Geometry: final body of the model. Coordinates: model frame, mm. Face numbers are marked on the shaded views. A direction names the side the tool comes from. Give positions to 0.01 mm unless a question says otherwise; leave off trailing zeros. Write each loop counter-clockwise with the first axis right and the second up, starting at its lowest first coordinate (ties: lowest second). Pieces come first, ordered by that corner, then holes. Notation, with made-up numbers: M 66,4 L 83,4 A9 ccw 83,17 Z; hole C 10,77 d9. An arc over 180 degrees is marked long. Use one line per item in the form item = value. Start each with the question number.
Item 1: Contact query for flat-ended pins moving along their axis: P1, Ø2.5, axis at x = -56.32, z = 56.54, coming from the -Y side; P2, Ø1, axis at x = -64.5, y = -29.5, coming from the +Z side. Output: stop coordinate, or through.
Item 2: Material intervals for line 1 along Y through (x, z) = (135, 71); line 2 along X through (y, z) = (17, 30.5) (3 decimals); line 3 along X through (y, z) = (-76.5, 37) (3 decimals), sorted ascending. Write a range as from..to.
Item 3: Section query D-D on x = -80.5. Return loops of the section in (y, z), then the cut area to 3 significant figures.
Item 4: Pull-direction query (X, two-part tool) for the marked faces 1, 2, 3 and 4; classes: released by +X, released by -X, zero draft, split by the parting line, or undercut.
Item 5: Access query for the marked faces 5 and 6. Directions: +Z, -Z, +X, -X, +Y, -Y. A direction counts if a zero-diameter tool reaches every point of the face in a straight line with its end or side. Return the directions, or none.
Item 6: Section query B-B on z = 113. Return loops of the section in (x, y) (3 decimals).
Item 7: Section query A-A on x = 25. Return loops of the section in (y, z), then the cut area to 3 significant figures.
Item 8: Section query C-C on y = -97. Return loops of the section in (x, z) (3 decimals).
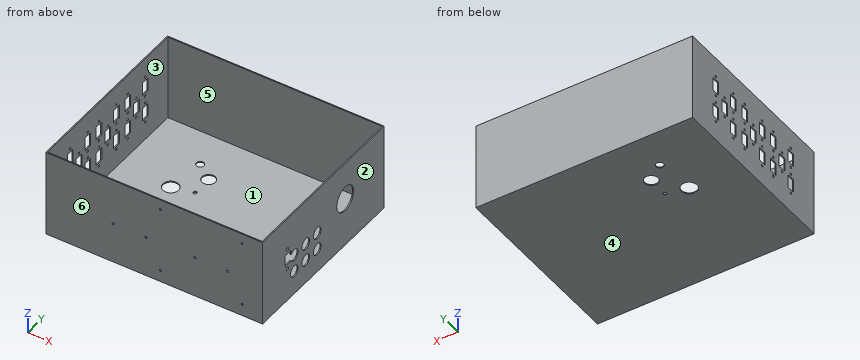
from build123d import *

# Parameters (mm, degrees)
SKETCH2_W                        = 298.45
SKETCH2_H                        = 254
BOSS_EXTRUDE1_DEPTH              = 120.65
SHELL1_T                         = -1.5
PT_CONNECTOR_CUTOUTS_REACH       = 348.06
SKETCH3_R                        = 8
SKETCH4_R                        = 1.55
SKETCH4_W                        = 18.7
SKETCH4_H                        = 11.8
SOLENOID_CONNECTOR_CUTOUTS_DEPTH = 1.5
SKETCH5_R                        = 1.524
PCB_MOUNTING_HOLES_DEPTH         = 1.5
SKETCH6_R                        = 17.574098895
CUT_EXTRUDE2_DEPTH               = 1.5
SKETCH7_R                        = 10.735729294
SKETCH7_R_2                      = 9.212667567
SKETCH7_R_3                      = 5.203861924
SKETCH7_R_4                      = 2.440691802
CUT_EXTRUDE3_DEPTH               = 1.5
SKETCH8_R                        = 2.06375
SKETCH8_W                        = 15.748
SKETCH8_H                        = 13.081
CUT_EXTRUDE4_DEPTH               = 1.5


with BuildPart() as part:
    # Sketch2 → Boss-Extrude1 (new body)
    with BuildSketch(Plane.XY):
        Rectangle(SKETCH2_W, SKETCH2_H)
    extrude(amount=BOSS_EXTRUDE1_DEPTH)

    # Shell1
    shell1_openings = [part.faces().sort_by_distance(p)[0] for p in [
        (0, 0, 120.65),
    ]]
    offset(amount=SHELL1_T, openings=shell1_openings, kind=Kind.INTERSECTION)

    # Sketch3 → PT Connector Cutouts (cut, up to next)
    with BuildSketch(Plane(origin=(149.225, 0, 0), x_dir=(0, 0, -1), z_dir=(1, 0, 0)), mode=Mode.PRIVATE) as pt_connector_cutouts_sk1:
        with Locations((-57.239729717, -60.69208043)):
            Circle(SKETCH3_R)
    pt_connector_cutouts_tool1 = extrude(pt_connector_cutouts_sk1.sketch, amount=-PT_CONNECTOR_CUTOUTS_REACH, mode=Mode.PRIVATE) & part.part
    # Sketch3 → PT Connector Cutouts (cut, up to next)
    with BuildSketch(Plane(origin=(149.225, 0, 0), x_dir=(0, 0, -1), z_dir=(1, 0, 0)), mode=Mode.PRIVATE) as pt_connector_cutouts_sk2:
        with Locations((-33.239729717, -60.69208043)):
            Circle(SKETCH3_R)
    pt_connector_cutouts_tool2 = extrude(pt_connector_cutouts_sk2.sketch, amount=-PT_CONNECTOR_CUTOUTS_REACH, mode=Mode.PRIVATE) & part.part
    # Sketch3 → PT Connector Cutouts (cut, up to next)
    with BuildSketch(Plane(origin=(149.225, 0, 0), x_dir=(0, 0, -1), z_dir=(1, 0, 0)), mode=Mode.PRIVATE) as pt_connector_cutouts_sk3:
        with Locations((-33.239729717, -36.69208043)):
            Circle(SKETCH3_R)
    pt_connector_cutouts_tool3 = extrude(pt_connector_cutouts_sk3.sketch, amount=-PT_CONNECTOR_CUTOUTS_REACH, mode=Mode.PRIVATE) & part.part
    # Sketch3 → PT Connector Cutouts (cut, up to next)
    with BuildSketch(Plane(origin=(149.225, 0, 0), x_dir=(0, 0, -1), z_dir=(1, 0, 0)), mode=Mode.PRIVATE) as pt_connector_cutouts_sk4:
        with Locations((-33.239729717, -12.69208043)):
            Circle(SKETCH3_R)
    pt_connector_cutouts_tool4 = extrude(pt_connector_cutouts_sk4.sketch, amount=-PT_CONNECTOR_CUTOUTS_REACH, mode=Mode.PRIVATE) & part.part
    # Sketch3 → PT Connector Cutouts (cut, up to next)
    with BuildSketch(Plane(origin=(149.225, 0, 0), x_dir=(0, 0, -1), z_dir=(1, 0, 0)), mode=Mode.PRIVATE) as pt_connector_cutouts_sk5:
        with Locations((-57.239729717, -36.69208043)):
            Circle(SKETCH3_R)
    pt_connector_cutouts_tool5 = extrude(pt_connector_cutouts_sk5.sketch, amount=-PT_CONNECTOR_CUTOUTS_REACH, mode=Mode.PRIVATE) & part.part
    # Sketch3 → PT Connector Cutouts (cut, up to next)
    with BuildSketch(Plane(origin=(149.225, 0, 0), x_dir=(0, 0, -1), z_dir=(1, 0, 0)), mode=Mode.PRIVATE) as pt_connector_cutouts_sk6:
        with Locations((-57.239729717, -12.69208043)):
            Circle(SKETCH3_R)
    pt_connector_cutouts_tool6 = extrude(pt_connector_cutouts_sk6.sketch, amount=-PT_CONNECTOR_CUTOUTS_REACH, mode=Mode.PRIVATE) & part.part
    add(pt_connector_cutouts_tool1.solids().sort_by_distance((149.225, -60.69208, 57.23973))[0], mode=Mode.SUBTRACT)
    add(pt_connector_cutouts_tool2.solids().sort_by_distance((149.225, -60.69208, 33.23973))[0], mode=Mode.SUBTRACT)
    add(pt_connector_cutouts_tool3.solids().sort_by_distance((149.225, -36.69208, 33.23973))[0], mode=Mode.SUBTRACT)
    add(pt_connector_cutouts_tool4.solids().sort_by_distance((149.225, -12.69208, 33.23973))[0], mode=Mode.SUBTRACT)
    add(pt_connector_cutouts_tool5.solids().sort_by_distance((149.225, -36.69208, 57.23973))[0], mode=Mode.SUBTRACT)
    add(pt_connector_cutouts_tool6.solids().sort_by_distance((149.225, -12.69208, 57.23973))[0], mode=Mode.SUBTRACT)

    # Sketch4 → Solenoid Connector Cutouts (cut)
    with BuildSketch(Plane.ZY.offset(149.225)):
        with Locations(Location((55.387501773, 78.156254231, 0), (0, 0, 270))):
            Circle(SKETCH4_R)
        with Locations(Location((27.162501773, 78.156254231, 0), (0, 0, 90))):
            Circle(SKETCH4_R)
        with Locations(Location((93.487501773, 78.156254231, 0), (0, 0, 270))):
            Circle(SKETCH4_R)
        with Locations(Location((65.262501773, 78.156254231, 0), (0, 0, 90))):
            Circle(SKETCH4_R)
        with Locations(Location((93.487501773, 41.643754231, 0), (0, 0, 270))):
            Circle(SKETCH4_R)
        with Locations(Location((65.262501773, 41.643754231, 0), (0, 0, 90))):
            Circle(SKETCH4_R)
        with Locations(Location((93.487501773, 18.256254231, 0), (0, 0, 270))):
            Circle(SKETCH4_R)
        with Locations(Location((65.262501773, 18.256254231, 0), (0, 0, 90))):
            Circle(SKETCH4_R)
        with Locations(Location((93.487501773, -18.256245769, 0), (0, 0, 270))):
            Circle(SKETCH4_R)
        with Locations(Location((65.262501773, -18.256245769, 0), (0, 0, 90))):
            Circle(SKETCH4_R)
        with Locations(Location((93.487501773, -41.643745769, 0), (0, 0, 270))):
            Circle(SKETCH4_R)
        with Locations(Location((65.262501773, -41.643745769, 0), (0, 0, 90))):
            Circle(SKETCH4_R)
        with Locations(Location((93.487501773, -78.156245769, 0), (0, 0, 270))):
            Circle(SKETCH4_R)
        with Locations(Location((65.262501773, -78.156245769, 0), (0, 0, 90))):
            Circle(SKETCH4_R)
        with Locations(Location((74.437501773, 59.900004231, 0), (0, 0, 270))):
            Circle(SKETCH4_R)
        with Locations(Location((46.212501773, 59.900004231, 0), (0, 0, 90))):
            Circle(SKETCH4_R)
        with Locations(Location((55.387501773, 41.643754231, 0), (0, 0, 270))):
            Circle(SKETCH4_R)
        with Locations(Location((27.162501773, 41.643754231, 0), (0, 0, 90))):
            Circle(SKETCH4_R)
        with Locations(Location((55.387501773, 18.256254231, 0), (0, 0, 270))):
            Circle(SKETCH4_R)
        with Locations(Location((27.162501773, 18.256254231, 0), (0, 0, 90))):
            Circle(SKETCH4_R)
        with Locations(Location((74.437501773, 4.231e-06, 0), (0, 0, 270))):
            Circle(SKETCH4_R)
        with Locations(Location((46.212501773, 4.231e-06, 0), (0, 0, 90))):
            Circle(SKETCH4_R)
        with Locations(Location((55.387501773, -18.256245769, 0), (0, 0, 270))):
            Circle(SKETCH4_R)
        with Locations(Location((27.162501773, -18.256245769, 0), (0, 0, 90))):
            Circle(SKETCH4_R)
        with Locations(Location((55.387501773, -41.643745769, 0), (0, 0, 270))):
            Circle(SKETCH4_R)
        with Locations(Location((27.162501773, -41.643745769, 0), (0, 0, 90))):
            Circle(SKETCH4_R)
        with Locations(Location((74.437501773, -59.899995769, 0), (0, 0, 270))):
            Circle(SKETCH4_R)
        with Locations(Location((46.212501773, -59.899995769, 0), (0, 0, 90))):
            Circle(SKETCH4_R)
        with Locations(Location((55.387501773, -78.156245769, 0), (0, 0, 270))):
            Circle(SKETCH4_R)
        with Locations(Location((27.162501773, -78.156245769, 0), (0, 0, 90))):
            Circle(SKETCH4_R)
        with Locations((41.275001773, 78.156254231)):
            Rectangle(SKETCH4_W, SKETCH4_H)
        with Locations((79.375001773, 78.156254231)):
            Rectangle(SKETCH4_W, SKETCH4_H)
        with Locations((79.375001773, 41.643754231)):
            Rectangle(SKETCH4_W, SKETCH4_H)
        with Locations((79.375001773, 18.256254231)):
            Rectangle(SKETCH4_W, SKETCH4_H)
        with Locations((79.375001773, -18.256245769)):
            Rectangle(SKETCH4_W, SKETCH4_H)
        with Locations((79.375001773, -41.643745769)):
            Rectangle(SKETCH4_W, SKETCH4_H)
        with Locations((79.375001773, -78.156245769)):
            Rectangle(SKETCH4_W, SKETCH4_H)
        with Locations((60.325001773, 59.900004231)):
            Rectangle(SKETCH4_W, SKETCH4_H)
        with Locations((41.275001773, 41.643754231)):
            Rectangle(SKETCH4_W, SKETCH4_H)
        with Locations((41.275001773, 18.256254231)):
            Rectangle(SKETCH4_W, SKETCH4_H)
        with Locations((60.325001773, 4.231e-06)):
            Rectangle(SKETCH4_W, SKETCH4_H)
        with Locations((41.275001773, -18.256245769)):
            Rectangle(SKETCH4_W, SKETCH4_H)
        with Locations((41.275001773, -41.643745769)):
            Rectangle(SKETCH4_W, SKETCH4_H)
        with Locations((60.325001773, -59.899995769)):
            Rectangle(SKETCH4_W, SKETCH4_H)
        with Locations((41.275001773, -78.156245769)):
            Rectangle(SKETCH4_W, SKETCH4_H)
    extrude(amount=-SOLENOID_CONNECTOR_CUTOUTS_DEPTH, mode=Mode.SUBTRACT)

    # Sketch5 → PCB Mounting Holes (cut)
    with BuildSketch(Plane(origin=(0, -127, 127), x_dir=(-1, 0, 0), z_dir=(0, 1, 0))):
        with Locations(Location((-121.235859114, -20.462314931, 0), (0, 0, 270))):
            Circle(SKETCH5_R)
        with Locations(Location((-56.235859114, -70.462314931, 0), (0, 0, 270))):
            Circle(SKETCH5_R)
        with Locations(Location((-121.235859114, -110.462314931, 0), (0, 0, 270))):
            Circle(SKETCH5_R)
        with Locations(Location((-101.235859114, -70.462314931, 0), (0, 0, 270))):
            Circle(SKETCH5_R)
        with Locations(Location((-8.675032002, -20.462314931, 0), (0, 0, 270))):
            Circle(SKETCH5_R)
        with Locations(Location((56.324967998, -70.462314931, 0), (0, 0, 270))):
            Circle(SKETCH5_R)
        with Locations(Location((-8.675032002, -110.462314931, 0), (0, 0, 270))):
            Circle(SKETCH5_R)
        with Locations(Location((11.324967998, -70.462314931, 0), (0, 0, 270))):
            Circle(SKETCH5_R)
    extrude(amount=PCB_MOUNTING_HOLES_DEPTH, mode=Mode.SUBTRACT)

    # Sketch6 → Cut-Extrude2 (cut)
    with BuildSketch(Plane(origin=(149.225, 0, 0), x_dir=(0, 0, -1), z_dir=(1, 0, 0))):
        with Locations((-68.387091128, 45.43625367)):
            Circle(SKETCH6_R)
    extrude(amount=-CUT_EXTRUDE2_DEPTH, mode=Mode.SUBTRACT)

    # Sketch7 → Cut-Extrude3 (cut)
    with BuildSketch(Plane(origin=(0, 0, 0), x_dir=(-1, 0, 0), z_dir=(0, 0, -1))):
        with Locations((75.19126283, 21.756760288)):
            Circle(SKETCH7_R)
        with Locations((46.368160054, 57.132321186)):
            Circle(SKETCH7_R_2)
        with Locations((69.95079545, 74.993212306)):
            Circle(SKETCH7_R_3)
        with Locations((46.368160054, 28.685666471)):
            Circle(SKETCH7_R_4)
    extrude(amount=-CUT_EXTRUDE3_DEPTH, mode=Mode.SUBTRACT)

    # Sketch8 → Cut-Extrude4 (cut)
    with BuildSketch(Plane.ZY.offset(-149.225)):
        with Locations((46.52594904, -74.819755611)):
            Circle(SKETCH8_R)
        with Locations(Location((75.35494904, -74.819755611, 0), (0, 0, 180))):
            Circle(SKETCH8_R)
        with Locations((60.94044904, -73.691658038)):
            Rectangle(SKETCH8_W, SKETCH8_H)
    extrude(amount=CUT_EXTRUDE4_DEPTH, mode=Mode.SUBTRACT)


solid = part.part
Answer sheet:
q1.P1 = 125.5
q1.P2 = 1.5
q2.line_1 = -127..-125.5, 125.5..127
q2.line_2 = -149.225..-147.725, 147.725..149.225
q2.line_3 = 147.725..149.225
q3.outline = M -127,0 L 12.43,0 L 12.43,1.5 L -125.5,1.5 L -125.5,120.65 L -127,120.65 Z; M 31.09,0 L 127,0 L 127,120.65 L 125.5,120.65 L 125.5,1.5 L 31.09,1.5 Z
q3.area = 710 mm2
q4.face_1 = undercut
q4.face_2 = released by +X
q4.face_3 = undercut
q4.face_4 = zero draft
q5.face_5 = +Z
q5.face_6 = +Z, -Z, +X, -X, -Y
q6.outline = M -149.225,-127 L 149.225,-127 L 149.225,127 L -149.225,127 Z; hole M -147.725,-125.5 L 147.725,-125.5 L 147.725,125.5 L -147.725,125.5 Z
q7.outline = M -127,0 L 127,0 L 127,120.65 L 125.5,120.65 L 125.5,1.5 L -125.5,1.5 L -125.5,120.65 L -127,120.65 Z
q7.area = 738 mm2
q8.outline = M -149.225,0 L 149.225,0 L 149.225,120.65 L 147.725,120.65 L 147.725,1.5 L -147.725,1.5 L -147.725,120.65 L -149.225,120.65 Z
